```python
from build123d import *

# Parameters (mm, degrees)
PAD_DEPTH       = 4
SKETCH001_R     = 1.5
POCKET_DEPTH    = 4.001
POCKET001_DEPTH = 4.001
SKETCH003_R     = 3
POCKET002_DEPTH = 2


with BuildPart() as part:
    # Sketch → Pad (new body)
    with BuildSketch(Plane.XZ):
        Polygon((16, 0), (16, -27.2), (0, -27.2), (0, 0), (-11.5, 0), (-11.5, 5), (20, 5), (20, 0), align=None)
    extrude(amount=PAD_DEPTH)

    # Sketch001 (on Face10 of Pad) → Pocket (cut, through all)
    with BuildSketch(Plane.XZ.offset(4)):
        with Locations((-3.625, 2.5)):
            Circle(SKETCH001_R)
        with Locations((4.25, 2.5)):
            Circle(SKETCH001_R)
        with Locations((12.125, 2.5)):
            Circle(SKETCH001_R)
    extrude(amount=-POCKET_DEPTH, mode=Mode.SUBTRACT)

    # Sketch002 (on Face5 of Pocket) → Pocket001 (cut, through all)
    with BuildSketch(Plane.XZ.offset(4)):
        with BuildLine():
            ThreePointArc((9.55, -5), (8, -3.45), (6.45, -5))
            Line((6.45, -5), (6.45, -8))
            ThreePointArc((6.45, -8), (8, -9.55), (9.55, -8))
            Line((9.55, -8), (9.55, -5))
        make_face()
        with BuildLine():
            ThreePointArc((9.55, -21), (8, -19.45), (6.45, -21))
            Line((6.45, -21), (6.45, -24))
            ThreePointArc((6.45, -24), (8, -25.55), (9.55, -24))
            Line((9.55, -24), (9.55, -21))
        make_face()
    extrude(amount=-POCKET001_DEPTH, mode=Mode.SUBTRACT)

    # Sketch003 (on Face5 of Pocket001) → Pocket002 (cut)
    with BuildSketch(Plane.XZ.offset(4)):
        with Locations((-3.625, 2.5)):
            Circle(SKETCH003_R)
        with Locations((4.25, 2.5)):
            Circle(SKETCH003_R)
        with Locations((12.125, 2.5)):
            Circle(SKETCH003_R)
        with BuildLine():
            ThreePointArc((11.05, -5), (8, -1.95), (4.95, -5))
            Line((4.95, -5), (4.95, -8))
            ThreePointArc((4.95, -8), (8, -11.05), (11.05, -8))
            Line((11.05, -8), (11.05, -5))
        make_face()
        with BuildLine():
            ThreePointArc((11.05, -21), (8, -17.95), (4.95, -21))
            Line((4.95, -21), (4.95, -24))
            ThreePointArc((4.95, -24), (8, -27.05), (11.05, -24))
            Line((11.05, -24), (11.05, -21))
        make_face()
    extrude(amount=-POCKET002_DEPTH, mode=Mode.SUBTRACT)


solid = part.part
```
Here's how the part is built. I have some questions about the finished solid (model axes, mm). A direction names the side the tool comes from. Coordinates: 2 decimals unless noted, no trailing zeros. Loops run counter-clockwise (first coordinate to the right, second up) from the corner with the lowest first, then second, coordinate; pieces in that order, holes last. Notation, with made-up numbers: (-38.5, 30) -> (2.5, 30) arc R15 ccw to (2.5, 42) -> close; hole circle Ø4 at (-9, -5.75). An arc over 180 degrees is marked (long way). Return JSON: item names as keys, results as strings.
1) If we section it at A-A, the plane x = 8: Write out the boundary of the cut face in (y, z), then the cut area to 3 significant figures.
Results below:
{"outline": "(-4, -27.2) -> (0, -27.2) -> (0, -25.55) -> (-2, -25.55) -> (-2, -27.05) -> (-4, -27.05) -> close; (-4, -17.95) -> (-2, -17.95) -> (-2, -19.45) -> (0, -19.45) -> (0, -9.55) -> (-2, -9.55) -> (-2, -11.05) -> (-4, -11.05) -> close; (-4, -1.95) -> (-2, -1.95) -> (-2, -3.45) -> (0, -3.45) -> (0, 5) -> (-4, 5) -> close", "area": "68.0 mm²"}
2) I need wall thicknesses on line 1 (X direction, y = -3.1, z = 2.5) (3 decimals); line 2 (X direction, y = -1, z = -6.5); line 3 (Z direction, x = 5.5, y = -3.35). Which ranges of each line are inside material? Lowest first, please. Write a range as from..to.
Results below:
{"line 1": "-11.5..-6.625, -0.625..1.25, 7.25..9.125, 15.125..20", "line 2": "0..6.45, 9.55..16", "line 3": "-27.2..-25.75, -19.25..-9.75, -3.25..-0.23"}
3) If we section it at D-D, the plane y = -1.6: Write out the boundary of the cut face in (x, z) (3 decimals), then the cut area to 3 significant figures.
Results below:
{"outline": "(-11.5, 0) -> (0, 0) -> (0, -27.2) -> (16, -27.2) -> (16, 0) -> (20, 0) -> (20, 5) -> (-11.5, 5) -> close; hole circle Ø3 at (-3.625, 2.5); hole circle Ø3 at (4.25, 2.5); hole (6.45, -24) arc R1.55 ccw to (9.55, -24) -> (9.55, -21) arc R1.55 ccw to (6.45, -21) -> close; hole (6.45, -8) arc R1.55 ccw to (9.55, -8) -> (9.55, -5) arc R1.55 ccw to (6.45, -5) -> close; hole circle Ø3 at (12.125, 2.5)", "area": "538 mm²"}
4) If we section it at B-B, the plane x = 4.25: Write out the boundary of the cut face in (y, z), then the cut area to 3 significant figures.
Results below:
{"outline": "(-4, -27.2) -> (0, -27.2) -> (0, 1) -> (-2, 1) -> (-2, -0.5) -> (-4, -0.5) -> close; (-2, 4) -> (0, 4) -> (0, 5) -> (-2, 5) -> close", "area": "112 mm²"}
5) For faces 4 (the face through (16, -2, -13)), 5 (the face through (6.45, -1, -6)), 6 (the face through (7.93, -3.01, -11.05)), which set-ups out of +Z, -Z, +X, -X, +Y, -Y let a thin tool reach every point of the face, with its end or its side?
Results below:
{"face 4": "-Z, +X, +Y, -Y", "face 5": "+Y, -Y", "face 6": "-Y"}
6) If we section it at C-C, the plane z = -6.5: Write out the boundary of the cut face in (x, y), then the cut area to 3 significant figures.
Results below:
{"outline": "(0, -4) -> (4.95, -4) -> (4.95, -2) -> (6.45, -2) -> (6.45, 0) -> (0, 0) -> close; (9.55, -2) -> (11.05, -2) -> (11.05, -4) -> (16, -4) -> (16, 0) -> (9.55, 0) -> close", "area": "45.6 mm²"}
7) Will these pins go through, and if not, where does the flat tip stop? pin 1 (1.2 mm diameter, centred on x = 17, y = -2.5, fed in from -Z); pin 2 (6.5 mm diameter, centred on x = 8.5, z = -21, fed in from -Y); pin 3 (3 mm diameter, centred on x = 12, z = 3.5, fed in from -Y); pin 4 (0.6 mm diameter, centred on y = -3.5, z = -7, fed in from +X).
Results below:
{"pin 1": "z = 0", "pin 2": "y = -4", "pin 3": "y = -2", "pin 4": "x = 16"}
8) Thinking about a two-plate mould opening in X: for faces 1 (the face through (4, -1.5, 5)), 2 (the face through (20, -2, 3)), 3 (the face through (-6.625, -3.014, 2.541)), which applies, +X half, -X half, draft (parallel to the pull), parting line (faces both ways), or undercut?
Results below:
{"face 1": "draft", "face 2": "+X half", "face 3": "undercut"}
